The model under review builds one solid part; all positions refer to its coordinate system, in mm. Face numbers are marked on the shaded views. Round coordinates to 2 decimals unless told otherwise and drop trailing zeros. Loops run counter-clockwise (first coordinate to the right, second up) from the corner with the lowest first, then second, coordinate; pieces in that order, holes last. Notation, with made-up numbers: (-5.75, 88) -> (35.25, 88) arc R34 cw to (35.25, 125) -> close; hole circle Ø1 at (67, 54). An arc over 180 degrees is marked (long way). Write each question's results on one line, items separated by ' | '. Start each with the question number.
Item 1: We need section C-C (z = 0.45). Give the boundary of the cut face in (x, y) (3 decimals).
Item 2: For L1, parallel to Y at x = 0, z = 0.55 (3 decimals); L2, parallel to Z at x = -6.5, y = -11; L3, parallel to Y at x = 10, z = 0.1, list the stretches that pass through material, from the lowest coordinate up. Write a range as from..to.
Item 3: We need section A-A (y = 0). Give the boundary of the cut face in (x, z) (3 decimals).
Item 4: Mouldability with a two-part tool opening along Y and no side actions: class the marked faces 1 and 2 as pulls with the +Y half, pulls with the -Y half, needs draft (parallel to the pull), parting line crosses it, or undercut.
Item 5: We need section D-D (y = -5). Give the boundary of the cut face in (x, z), and give its area (3 significant figures).
Item 6: We need section B-B (x = 0). Give the boundary of the cut face in (y, z) (3 decimals), and give its area (3 significant figures).
Item 7: Clearance check with flat-ended pins moving along their axes: pin 1 Ø3 at (x, y) = (12.5, -11) entering from -Z; pin 2 Ø1.1 at (x, z) = (-13.5, 0.5) entering from -Y; pin 3 Ø0.8 at (x, z) = (-11.5, -2) entering from -Y. State where each tip first meets the part, or that it passes through.
from build123d import *

# Parameters (mm, degrees)
SKETCH1_R                    = 7.715
BASE_FLANGE1_DEPTH           = 1
EDGE_FLANGE1_STRIP_W         = 5
EDGE_FLANGE1_STRIP_H         = 1
EDGE_FLANGE1_STRIP_CUT_DEPTH = 4.5
EDGE_FLANGE1_DEPTH           = 4.5


# Sheet-metal steps are written as plain solids
with BuildPart() as part:
    # Sketch1 → Base-Flange1 (new body)
    with BuildSketch(Plane.XY):
        with BuildLine():
            Line((-15.841006912, 2.25), (-12, 2.25))
            Line((-12, 2.25), (-12, -2.25))
            Line((-12, -2.25), (-15.841006912, -2.25))
            ThreePointArc((-15.841006912, -2.25), (16, 0), (-15.841006912, 2.25))
        make_face()
        Circle(SKETCH1_R, mode=Mode.SUBTRACT)
    extrude(amount=BASE_FLANGE1_DEPTH)

    # Edge-Flange1 strip (across the edge) → Edge-Flange1 strip cut (cut)
    with BuildSketch(Plane(origin=(-12, -2.25, 0), x_dir=(1, 0, 0), z_dir=(0, 1, 0))):
        with Locations((-1, -0.5)):
            Rectangle(EDGE_FLANGE1_STRIP_W, EDGE_FLANGE1_STRIP_H)
    extrude(amount=EDGE_FLANGE1_STRIP_CUT_DEPTH, mode=Mode.SUBTRACT)

    # Edge-Flange1 section (across the edge) → Edge-Flange1 (add)
    with BuildSketch(Plane(origin=(-12, -2.25, 0), x_dir=(1, 0, 0), z_dir=(0, 1, 0))):
        with BuildLine():
            Line((0, 0.5), (0, 3))
            Line((0, 3), (1, 3))
            Line((1, 3), (1, 0.5))
            ThreePointArc((1, 0.5), (1.146446609, 0.146446609), (1.5, 0))
            Line((1.5, 0), (1.5, -1))
            ThreePointArc((1.5, -1), (0.439339828, -0.560660172), (0, 0.5))
        make_face()
    extrude(amount=EDGE_FLANGE1_DEPTH)


solid = part.part
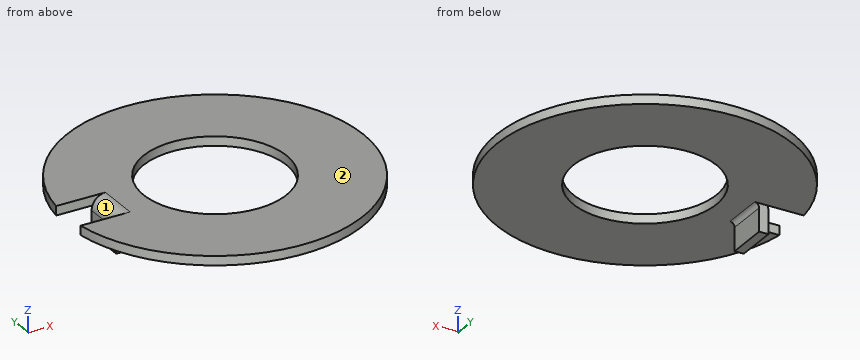
Here are the results:
1) outline: (-15.841, -2.25) arc R16 ccw (long way) to (-15.841, 2.25) -> (-11.661, 2.25) -> (-11.661, -2.25) -> close; hole circle Ø15.43 at (0, 0)
2) L1: y = -16..-7.715, 7.715..16 | L2: z = 0..1 | L3: y = -12.49..12.49
3) outline: (-12, -3) -> (-11, -3) -> (-11, -0.5) arc R0.5 cw to (-10.5, 0) -> (-7.715, 0) -> (-7.715, 1) -> (-10.5, 1) arc R1.5 ccw to (-12, -0.5) -> close; (7.715, 0) -> (16, 0) -> (16, 1) -> (7.715, 1) -> close
4) face 1: undercut | face 2: needs draft
5) outline: (-15.2, 0) -> (-5.88, 0) -> (-5.88, 1) -> (-15.2, 1) -> close; (5.88, 0) -> (15.2, 0) -> (15.2, 1) -> (5.88, 1) -> close | area: 18.6 mm2
6) outline: (-16, 0) -> (-7.715, 0) -> (-7.715, 1) -> (-16, 1) -> close; (7.715, 0) -> (16, 0) -> (16, 1) -> (7.715, 1) -> close | area: 16.6 mm2
7) pin 1: stops at z = 0 | pin 2: stops at y = -9.4 | pin 3: stops at y = -2.25
